Source: three-view drawing plus pictorial views. Frame: mm from the lowest corner of the part. A direction names the side the tool comes from. Round coordinates to 2 decimals unless told otherwise and drop trailing zeros. Loops run counter-clockwise (first coordinate to the right, second up) from the corner with the lowest first, then second, coordinate; pieces in that order, holes last. Notation, with made-up numbers: (79, 73.5) -> (116, 73.5) arc R21 cw to (116, 110.5) -> close; hole circle Ø11 at (39, 38.5). An arc over 180 degrees is marked (long way). Answer in a Markdown table with one row per item.
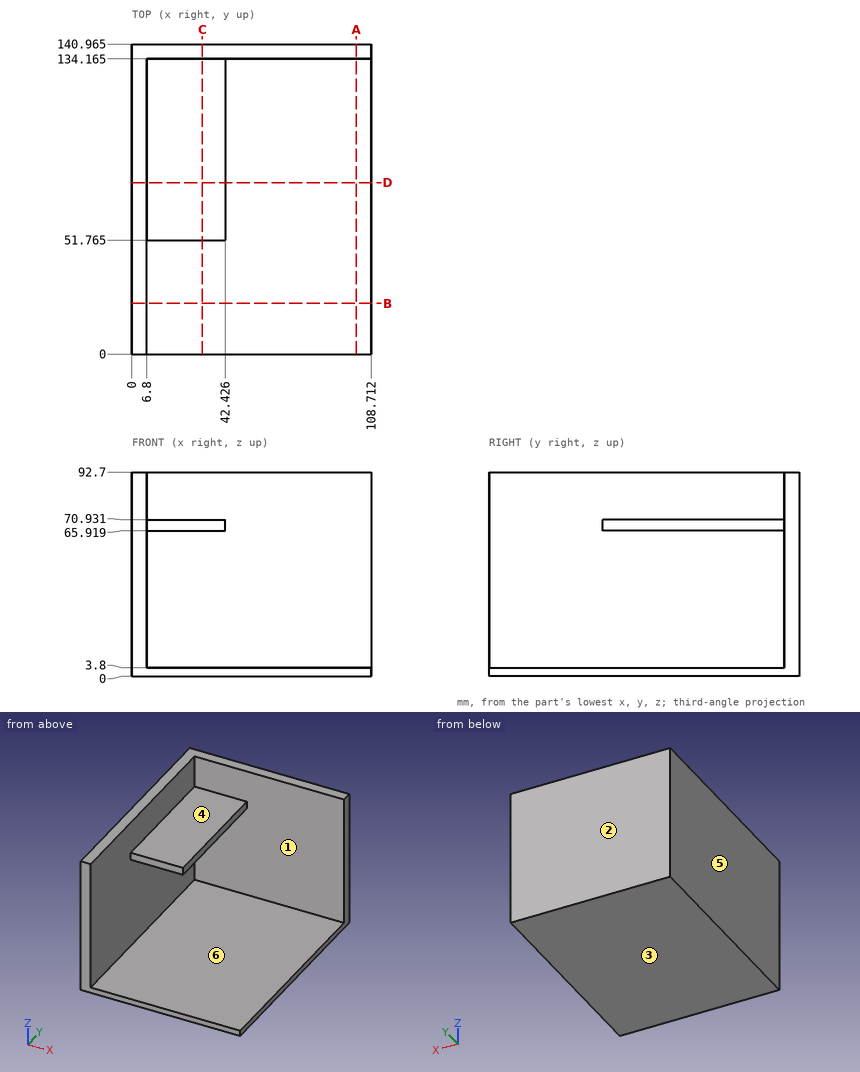
Item 1: Pin query (flat end, axial travel): pin 1 Ø6 at (x, z) = (45, 75.5) entering from -Y (1 decimal); pin 2 Ø18 at (x, y) = (28, 94) entering from +Z; pin 3 Ø8 at (y, z) = (78, 37) entering from +X. Return the tip coordinate at first contact, or that it passes through.
Answer:
| item | result |
|---|---|
| pin 1 | stops at y = 134.2 |
| pin 2 | stops at z = 70.93 |
| pin 3 | stops at x = 6.8 |
Item 2: Draft query along Z for the marked faces 1, 2 and 3. Return one class per face: pulls with the +Z half, pulls with the -Z half, needs draft (parallel to the pull), parting line crosses it, or undercut.
Answer:
| item | result |
|---|---|
| face 1 | undercut |
| face 2 | needs draft |
| face 3 | pulls with the -Z half |
Item 3: Reachability of the marked faces 4, 5 and 6 from +Z, -Z, +X, -X, +Y, -Y: full face, straight path, thin tool, end or side. Return the list, or none.
Answer:
| item | result |
|---|---|
| face 4 | +Z, +X, -Y |
| face 5 | +Z, -Z, -X, +Y, -Y |
| face 6 | +X, -Y |
Item 4: Cut plane C-C (x = 32). Output: boundary loops of the cut face in (y, z) (1 decimal).
Answer:
| item | result |
|---|---|
| outline | (0, 0) -> (141, 0) -> (141, 92.7) -> (134.2, 92.7) -> (134.2, 70.9) -> (51.8, 70.9) -> (51.8, 65.9) -> (134.2, 65.9) -> (134.2, 3.8) -> (0, 3.8) -> close |
Item 5: Cut plane A-A (x = 102). Output: boundary loops of the cut face in (y, z) (1 decimal).
Answer:
| item | result |
|---|---|
| outline | (0, 0) -> (141, 0) -> (141, 92.7) -> (134.2, 92.7) -> (134.2, 3.8) -> (0, 3.8) -> close |
Item 6: Line query: probe 1 along Z at (x, y) = (33.5, 59.5); probe 2 along Z at (x, y) = (51, 106); probe 3 along Y at (x, z) = (80, 39) (1 decimal). Output: solid intervals per line, ascending. Write a range as [from, to].
Answer:
| item | result |
|---|---|
| probe 1 | z = [0, 3.8], [65.92, 70.93] |
| probe 2 | z = [0, 3.8] |
| probe 3 | y = [134.2, 141] |
Item 7: Cut plane B-B (y = 23). Output: boundary loops of the cut face in (x, z), then the cut area to 3 significant figures.
Answer:
| item | result |
|---|---|
| outline | (0, 0) -> (108.71, 0) -> (108.71, 3.8) -> (6.8, 3.8) -> (6.8, 92.7) -> (0, 92.7) -> close |
| area | 1,020 mm² |
Item 8: Cut plane D-D (y = 78). Output: boundary loops of the cut face in (x, z) (1 decimal), then the cut area to 3 significant figures.
Answer:
| item | result |
|---|---|
| outline | (0, 0) -> (108.7, 0) -> (108.7, 3.8) -> (6.8, 3.8) -> (6.8, 65.9) -> (42.4, 65.9) -> (42.4, 70.9) -> (6.8, 70.9) -> (6.8, 92.7) -> (0, 92.7) -> close |
| area | 1,200 mm² |
